Part print with two shaded views. Sizes in mm from the minimum x, y, z corner. Give positions to 0.01 mm unless a question says otherwise; leave off trailing zeros. Order: outer loops, then holes, each group sorted by start corner. A loop starts at its lowest first (then second) coordinate and runs counter-clockwise, first axis right, second up. Notation, with made-up numbers: M 0.5,0.25 L 44.5,0.25 A23 cw 44.5,12.25 Z; hole C 34.25,-9 d11. An arc over 180 degrees is marked long. Return JSON: item names as keys, results as strings.
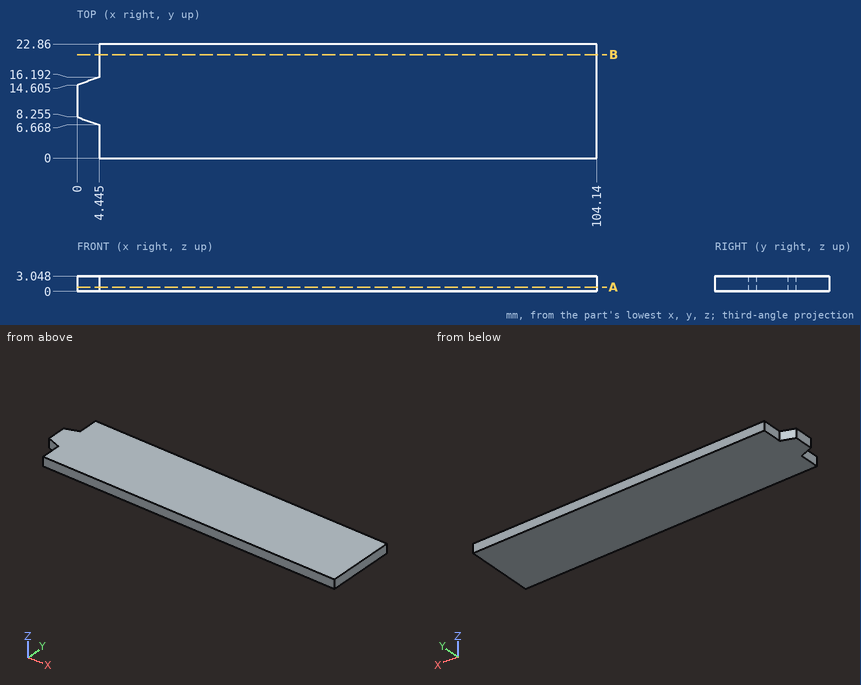
Q1. Band-saw the part on B-B (y = 20.75). Give the cut face in (x, z) (1 decimal), then the cut area to 3 significant figures.
Established:
{"outline": "M 4.4,0 L 104.1,0 L 104.1,3 L 4.4,3 Z", "area": "304 mm²"}
Q2. Pin check, flat tip, straight feed: pin 1 (0.9 mm diameter, centred on y = 4, z = 1, fed in from -X) (1 decimal). Stop position of the tip, or through.
Established:
{"pin 1": "stops at x = 4.4"}
Q3. Band-saw the part on A-A (z = 0.85). Give the cut face in (x, y) (1 decimal), then the cut area to 3 significant figures.
Established:
{"outline": "M 0,8.3 L 4.4,6.7 L 4.4,0 L 104.1,0 L 104.1,22.9 L 4.4,22.9 L 4.4,16.2 L 0,14.6 Z", "area": "2,310 mm²"}
Q4. Probe line 1 along X through (y, z) = (17, 2.1) (1 decimal). List the from-to ranges inside material, lowest first.
Established:
{"line 1": "x = 4.4 to 104.1"}
